CAD build for the part. Positions are in the model's coordinates, mm. Face numbers are marked on the shaded views. A direction names the side the tool comes from. Coordinates: 2 decimals unless noted, no trailing zeros. Loops run counter-clockwise (first coordinate to the right, second up) from the corner with the lowest first, then second, coordinate; pieces in that order, holes last. Notation, with made-up numbers: (25, -20) -> (30, -20) arc R37 cw to (30, 18) -> close; hole circle Ø8 at (-40, 83). An arc over 180 degrees is marked (long way). Write each question's results on one line, items separated by ' | '.
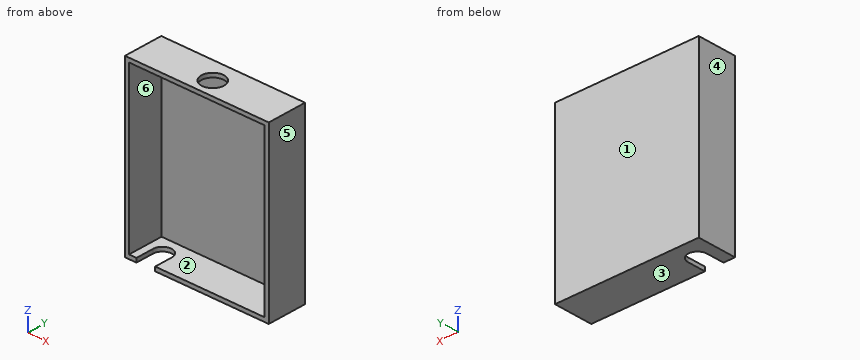
```python
from build123d import *

# Parameters (mm, degrees)
F0_W     = 31.7627
F0_H     = 76.454
F1_DEPTH = 16.51
F2_T     = 1.905
F3_R     = 5.2760492521
F4_DEPTH = 25.4
F5_R     = 4.3777369445
F6_DEPTH = 25.4
F9_DEPTH = 25.4


with BuildPart() as f1:
    # F0 (on Front) → F1 (new body)
    with BuildSketch(Plane.XZ):
        with Locations((15.88135, 8.247606141)):
            Rectangle(F0_W, F0_H)
        with Locations((-15.88135, 8.247606141)):
            Rectangle(F0_W, F0_H)
    extrude(amount=F1_DEPTH)

    # F2
    f2_openings = [f1.faces().sort_by_distance(p)[0] for p in [
        (0, -16.51, 8.247606),
    ]]
    offset(amount=F2_T, openings=f2_openings, kind=Kind.INTERSECTION)

    # F3 (on face) → F4 (cut)
    with BuildSketch(Plane.XY.offset(48.379606141)):
        with Locations((0, -8.4488391876)):
            Circle(F3_R)
    extrude(amount=-F4_DEPTH, mode=Mode.SUBTRACT)

    # F5 (on face) → F6 (cut)
    with BuildSketch(Plane(origin=(0, 0, -31.884393859), x_dir=(1, 0, 0), z_dir=(0, 0, -1))):
        with Locations((-23.9024627954, 8.0834906548)):
            Circle(F5_R)
    extrude(amount=-F6_DEPTH, mode=Mode.SUBTRACT)


with BuildPart() as f1_1:
    # F7: moved
    add(f1.part.moved(Location((0, 0, 31.115))))

    # F8 (on face) → F9 (cut)
    with BuildSketch(Plane(origin=(0, 0, -0.769393859), x_dir=(1, 0, 0), z_dir=(0, 0, -1))):
        Polygon((-28.2801996592, 8.0843311799), (-19.5247259315, 8.0843311799), (-19.5247259315, 16.51), (-28.2785819315, 16.51), align=None)
    extrude(amount=-F9_DEPTH, mode=Mode.SUBTRACT)


solid = f1_1.part
```
Q1. Cut at C-C on z = 11. Write the cut outline in (x, y) (3 decimals), and give its area (3 significant figures).
Results are:
outline: (-33.668, -16.51) -> (-31.763, -16.51) -> (-31.763, 0) -> (31.763, 0) -> (31.763, -16.51) -> (33.668, -16.51) -> (33.668, 1.905) -> (-33.668, 1.905) -> close | area: 191 mm^2
Q2. Cut at A-A on x = 0. Write the cut outline in (y, z) (3 decimals).
Results are:
outline: (-16.51, -0.769) -> (1.905, -0.769) -> (1.905, 79.495) -> (-3.173, 79.495) -> (-3.173, 77.59) -> (0, 77.59) -> (0, 1.136) -> (-16.51, 1.136) -> close; (-16.51, 77.59) -> (-13.725, 77.59) -> (-13.725, 79.495) -> (-16.51, 79.495) -> close
Q3. Which spindle directions (+Z, -Z, +X, -X, +Y, -Y) get a long thin tool onto all of the face, cutting with end or side? Do the marked faces 1 and 2. Say none if no direction does.
Results are:
face 1: +Z, -Z, +X, -X, +Y | face 2: -Y
Q4. Cut at B-B on y = -11.25. Write the cut outline in (x, z).
Results are:
outline: (-33.67, -0.77) -> (-28.28, -0.77) -> (-28.28, 1.14) -> (-31.76, 1.14) -> (-31.76, 77.59) -> (-4.47, 77.59) -> (-4.47, 79.49) -> (-33.67, 79.49) -> close; (-19.52, -0.77) -> (33.67, -0.77) -> (33.67, 79.49) -> (4.47, 79.49) -> (4.47, 77.59) -> (31.76, 77.59) -> (31.76, 1.14) -> (-19.52, 1.14) -> close
Q5. Wall check: L1, parallel to X at y = -6, z = 76; L2, parallel to Y at x = 0, z = 79.05 (3 decimals); L3, parallel to Z at x = -8, y = -11. Give the ranges that are in metal, low to high. Write a range as from..to.
Results are:
L1: -33.67..-31.76, 31.76..33.67 | L2: -16.51..-13.725, -3.173..1.905 | L3: -0.77..1.14, 77.59..79.49
Q6. Cut at D-D on x = 24.5. Write the cut outline in (y, z) (3 decimals).
Results are:
outline: (-16.51, -0.769) -> (1.905, -0.769) -> (1.905, 79.495) -> (-16.51, 79.495) -> (-16.51, 77.59) -> (0, 77.59) -> (0, 1.136) -> (-16.51, 1.136) -> close
Q7. Pull direction X, two halves, no side cores. Call the marked faces 3, 4, 5 and 6: +X half, -X half, draft (parallel to the pull), parting line (faces both ways), or undercut.
Results are:
face 3: draft | face 4: -X half | face 5: +X half | face 6: undercut
Q8. Drop a flat-ended pin along its axis: pin 1 (19 mm diameter, centred on x = 9, z = 27, fed in from -Y). Give the stop position or say it passes through.
Results are:
pin 1: y = 0
